Input: part model. Units: mm. Frame: model coordinates. A direction names the side the tool comes from. Give positions to 0.01 mm unless a question says otherwise; leave off trailing zeros. Order: outer loops, then holes, each group sorted by start corner. A loop starts at its lowest first (then second) coordinate and runs counter-clockwise, first axis right, second up. Notation, with made-up numbers: (79, 65.5) - (109, 65.5) arc R26 ccw to (109, 85.5) - close; hole circle Ø3 at (42.5, 29). An arc over 180 degrees is marked (long way). Use a Markdown table: item, result.
Autodesk Inventor part; units mm, degrees
ref_plane "YZ Plane" through (0, 0, 0) normal (1, 0, 0) x (0, 1, 0)
ref_plane "XZ Plane" through (0, 0, 0) normal (0, 1, 0) x (-1, 0, 0)
ref_plane "XY Plane" through (0, 0, 0) normal (0, 0, 1) x (1, 0, 0)
sketch "Sketch1" plane through (0, 0, 0) normal (0, 1, 0) x (-1, 0, 0)
  circle A0 centre (0, 0) radius 13.5
  dimension "d0" = 27
extrude "Extrusion1" add sketch "Sketch1" along normal blind 6
sketch "Sketch3" plane through (0, 6, 0) normal (0, 1, 0) x (1, 0, 0)
  point P0 (0, 0)
  point P1 (0, 0)
hole "Hole1" at (0, 6, 0) direction (0, -1, 0) diameter 8.5 end through all
sketch "Sketch4" plane through (0, 6, 0) normal (0, 1, 0) x (1, 0, 0)
  point P0 (0, 0)
  point P1 (-8.5, 0)
  point P2 (8.5, 0)
  dimension "d13" = 17
  dimension "d14" = 8.5
hole "Hole2" at (-8.5, 6, 0) at (8.5, 6, 0) direction (0, -1, 0) diameter 2.4 end through all counterbore diameter 4.4 counterbore depth 2.3
chamfer "Chamfer2" distance 0.5 angle 45 2 edges at (0, 0, -4.25) (0, 6, -4.25)
sketch "Sketch5" plane through (0, 6, 0) normal (0, 1, 0) x (1, 0, 0)
  line L0 (0, 0) -> (4, 12.8938) construction
  circle A0 centre (0, 0) radius 13.5 construction
  line L1 (0, 0) -> (-4, 12.8938) construction
  line L2 (0, 18.9) -> (0, -18.9) construction
  line L3 (4, 12.8938) -> (-4, 12.8938)
  arc A1 (4, 12.8938) -> (-4, 12.8938) centre (0, 0) ccw
  point P0 (0, 13.5)
  dimension "d28" = 8
extrude "Extrusion3" cut sketch "Sketch5" against normal through all
sketch "Sketch6" plane through (4, 6, -12.8938) normal (0, 0, -1) x (-1, 0, 0)
  line L0 (8, -6) -> (0, -6) construction
  line L1 (8, 0) -> (8, -6) construction
  line L2 (0, 0) -> (8, 0) construction
  line L3 (0, -6) -> (0, 0) construction
  line L4 (0, 0) -> (8, -6) construction
  point P0 (4, -6)
  point P1 (4, -3)
hole "Hole3" at (0, 3, -12.8938) direction (0, 0, 1) diameter 2.459 depth 10 tip angle 118
chamfer "Chamfer3" distance 0.2 angle 45 1 edges at (0, 1.7705, -12.8938)
properties part number "KN-00-02-12" material "CuZn40"
1. Section query A-A (z = 0). Return loops of the section in (x, y).
Response:
| item | result |
|---|---|
| outline | (-13.5, 0) - (-9.7, 0) - (-9.7, 3.7) - (-10.7, 3.7) - (-10.7, 6) - (-13.5, 6) - close; (-7.3, 0) - (-4.75, 0) - (-4.25, 0.5) - (-4.25, 5.5) - (-4.75, 6) - (-6.3, 6) - (-6.3, 3.7) - (-7.3, 3.7) - close; (4.25, 0.5) - (4.75, 0) - (7.3, 0) - (7.3, 3.7) - (6.3, 3.7) - (6.3, 6) - (4.75, 6) - (4.25, 5.5) - close; (9.7, 0) - (13.5, 0) - (13.5, 6) - (10.7, 6) - (10.7, 3.7) - (9.7, 3.7) - close |
2. Section query D-D (x = -8.5). Return loops of the section in (y, z), then the cut area to 3 significant figures.
Response:
| item | result |
|---|---|
| outline | (0, -10.49) - (6, -10.49) - (6, -2.2) - (3.7, -2.2) - (3.7, -1.2) - (0, -1.2) - close; (0, 1.2) - (3.7, 1.2) - (3.7, 2.2) - (6, 2.2) - (6, 10.49) - (0, 10.49) - close |
| area | 107 mm^2 |
3. Section query C-C (y = 3). Return loops of the section in (x, z), then the cut area to 3 significant figures.
Response:
| item | result |
|---|---|
| outline | (-4, -12.89) - (-1.43, -12.89) - (-1.23, -12.69) - (-1.23, -4.07) arc R4.25 cw (long way) to (1.23, -4.07) - (1.23, -12.69) - (1.43, -12.89) - (4, -12.89) arc R13.5 ccw (long way) to start; hole circle Ø2.4 at (-8.5, 0); hole circle Ø2.4 at (8.5, 0) |
| area | 482 mm^2 |
4. Material intervals for line 1 along X through (y, z) = (0.8, 0); line 2 along Y through (x, z) = (-9.75, -0.75); line 3 along Z through (x, y) = (3.25, 3.2), sorted ascending.
Response:
| item | result |
|---|---|
| line 1 | x = -13.5 to -9.7, -7.3 to -4.25, 4.25 to 7.3, 9.7 to 13.5 |
| line 2 | y = 0 to 3.7 |
| line 3 | z = -12.89 to -2.74, 2.74 to 13.1 |
5. Set-up query: faces 1 (the face through (0, 0, -5)), 2 (the face through (-10.355, 4.834, 1.183)). Return all of +Z, -Z, +X, -X, +Y, -Y with unobstructed straight access to the full face (end or side cutting, diameter ignored); none if empty.
Response:
| item | result |
|---|---|
| face 1 | +Z, -Z, +X, -X, -Y |
| face 2 | +Y |
6. Section query B-B (x = 0). Return loops of the section in (y, z).
Response:
| item | result |
|---|---|
| outline | (0, -12.89) - (1.57, -12.89) - (1.77, -12.69) - (1.77, -4.25) - (0.5, -4.25) - (0, -4.75) - close; (0, 4.75) - (0.5, 4.25) - (5.5, 4.25) - (6, 4.75) - (6, 13.5) - (0, 13.5) - close; (4.23, -12.69) - (4.43, -12.89) - (6, -12.89) - (6, -4.75) - (5.5, -4.25) - (4.23, -4.25) - close |
7. Mould query, pull axis Z, two halves, no side actions, for faces 3 (the face through (0.9, 4.4, -12.894)), 4 (the face through (-7.33, 1.82, -0.26)), 5 (the face through (1.09, 3.57, -8.32)). Classes: pulls with the +Z half, pulls with the -Z half, needs draft (parallel to the pull), parting line crosses it, or undercut.
Response:
| item | result |
|---|---|
| face 3 | pulls with the -Z half |
| face 4 | undercut |
| face 5 | needs draft |
8. Pin query (flat end, axial travel): pin 1 (8 mm diameter, centred on x = 8, z = -0.5, fed in from -Y); pin 2 (1 mm diameter, centred on x = -6, y = 1, fed in from +Z). Return the tip coordinate at first contact, or that it passes through.
Response:
| item | result |
|---|---|
| pin 1 | stops at y = 0 |
| pin 2 | stops at z = 12.33 |
